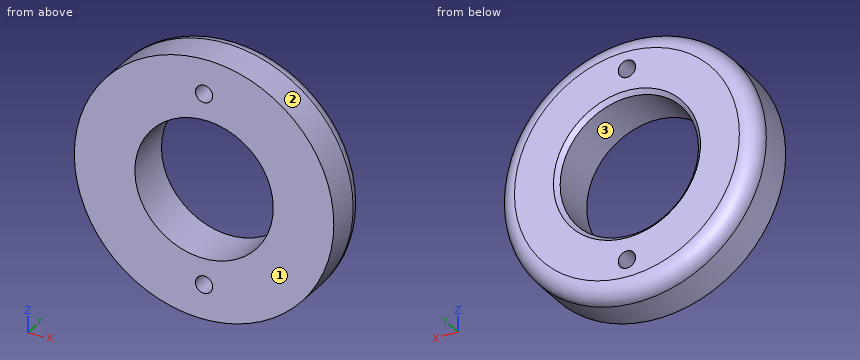
Autodesk Inventor part; units mm, degrees
ref_plane "YZ Plane" through (0, 0, 0) normal (1, 0, 0) x (0, 1, 0)
ref_plane "XZ Plane" through (0, 0, 0) normal (0, 1, 0) x (-1, 0, 0)
ref_plane "XY Plane" through (0, 0, 0) normal (0, 0, 1) x (1, 0, 0)
sketch "Boceto1" plane through (0, 0, 0) normal (0, 1, 0) x (-1, 0, 0)
  circle A0 centre (0, 0) radius 15
  dimension "d0" = 30
extrude "Extrusión1" add sketch "Boceto1" along normal blind 6
sketch "Boceto2" plane through (0, 0, 0) normal (0, -1, 0) x (1, 0, 0)
  circle A0 centre (0, 0) radius 8
  dimension "d3" = 16
extrude "Extrusión2" cut sketch "Boceto2" against normal through all
fillet "Empalme1" radius 2 1 edges at (15, 6, 0)
chamfer "Chaflán1" distance 0.5 angle 45 1 edges at (-8, 6, 0)
sketch "Boceto3" plane through (0, 6, 0) normal (0, 1, 0) x (1, 0, 0)
  circle A0 centre (0, 0) radius 13
  circle A1 centre (0, 0) radius 11 construction
  point P0 (0, 11)
  point P1 (0, -11)
  dimension "d10" = 2
hole "Agujero1" at (0, 6, -11) at (0, 6, 11) direction (0, -1, 0) diameter 2 end through all
properties part number "wheel_washer" material "Aluminio 6061"
Geometry: final body of the model. Coordinates: model frame, mm. Face numbers are marked on the shaded views. Round coordinates to 2 decimals unless told otherwise and drop trailing zeros. Loops run counter-clockwise (first coordinate to the right, second up) from the corner with the lowest first, then second, coordinate; pieces in that order, holes last. Notation, with made-up numbers: (1.25, 40.25) -> (19.25, 40.25) arc R30 ccw to (19.25, 75.25) -> close; hole circle Ø11 at (62.25, -38.75). An arc over 180 degrees is marked (long way). Use one line per item in the form item = value.
Item 1: Draft query along X for the marked faces 1, 2 and 3. Return one class per face: released by +X, released by -X, zero draft, split by the parting line, or undercut.
Evaluation:
face_1 = zero draft
face_2 = split by the parting line
face_3 = undercut
Item 2: Cut plane A-A on z = 0. Output: boundary loops of the cut face in (x, y), then the cut area to 3 significant figures.
Evaluation:
outline = (-15, 0) -> (-8, 0) -> (-8, 5.5) -> (-8.5, 6) -> (-13, 6) arc R2 ccw to (-15, 4) -> close; (8, 0) -> (15, 0) -> (15, 4) arc R2 ccw to (13, 6) -> (8.5, 6) -> (8, 5.5) -> close
area = 82.0 mm2
Item 3: Contact query for flat-ended pins moving along their axis: pin 1 Ø14.5 at (x, z) = (0, 0) entering from +Y; pin 2 Ø1 at (x, y) = (-1, 1.5) entering from +Z; pin 3 Ø3 at (y, z) = (0.5, -10.5) entering from -X. Output: stop coordinate, or through.
Evaluation:
pin_1 = through
pin_2 = 14.99
pin_3 = -12
Item 4: Material intervals for probe 1 along Z at (x, y) = (0, 3.3); probe 2 along X at (y, z) = (4.2, -11); probe 3 along X at (y, z) = (2, 10.5), sorted ascending.
Evaluation:
probe_1 = -15 to -12, -10 to -8, 8 to 10, 12 to 15
probe_2 = -10.18 to -1, 1 to 10.18
probe_3 = -10.71 to -0.87, 0.87 to 10.71
Item 5: Cut plane C-C on y = 4.85. Output: boundary loops of the cut face in (x, z), then the cut area to 3 significant figures.
Evaluation:
outline = circle Ø29.62 at (0, 0); hole circle Ø16 at (0, 0); hole circle Ø2 at (0, -11); hole circle Ø2 at (0, 11)
area = 482 mm2
Item 6: Cut plane B-B on y = 2.9. Output: boundary loops of the cut face in (x, z), then the cut area to 3 significant figures.
Evaluation:
outline = circle Ø30 at (0, 0); hole circle Ø16 at (0, 0); hole circle Ø2 at (0, -11); hole circle Ø2 at (0, 11)
area = 500 mm2
